Input: part model. Units: mm. Frame: model coordinates. Coordinates: 2 decimals unless noted, no trailing zeros. Order: outer loops, then holes, each group sorted by start corner. A loop starts at its lowest first (then second) coordinate and runs counter-clockwise, first axis right, second up. Notation, with made-up numbers: (-16, 7) -> (16, 7) arc R28 ccw to (16, 29) -> close; hole circle Ø1 at (83, 83). An arc over 180 degrees is marked (long way). One line per question, with ' | ' between items.
Autodesk Fusion 360 part; units mm, degrees
sketch "Sketch1" plane through (0, 0, 0) normal (0, 1, 0) x (1, 0, 0)
  circle A0 centre (0, 0) radius 1.55
  circle A1 centre (0, 0) radius 2.75
  line L0 (0, 2.75) -> (37, 2.75)
  line L1 (29.0028, 0) -> (29.0028, 0)
  line L2 (37, -2.75) -> (0, -2.75)
  arc A2 (39.75, 0) -> (37, 2.75) centre (37, 0) ccw
  arc A3 (37, -2.75) -> (39.75, 0) centre (37, 0) ccw
  dimension "d1" = 3.1
  dimension "d3" = 5.5
  dimension "d4" = 2.75
  dimension "d6" = 37
extrude "Extrude1" add sketch "Sketch1" along normal blind 2
equation "d6 = 40 mm - d4 - 0.25 mm"
1. Cut plane C-C, the plane z = 2. Return loops of the section in (x, y), and give its area (4 significant figures).
Recorded:
outline: (-1.89, 0) -> (38.89, 0) -> (38.89, 2) -> (-1.89, 2) -> close | area: 81.55 mm^2
2. Cut plane A-A, the plane z = 0. Return loops of the section in (x, y), and give its area (3 significant figures).
Recorded:
outline: (-2.75, 0) -> (-1.55, 0) -> (-1.55, 2) -> (-2.75, 2) -> close; (1.55, 0) -> (39.75, 0) -> (39.75, 2) -> (1.55, 2) -> close | area: 78.8 mm^2
3. Cut plane B-B, the plane y = 1.25. Return loops of the section in (x, z), and give its area (3 significant figures).
Recorded:
outline: (0, -2.75) -> (37, -2.75) arc R2.75 ccw to (37, 2.75) -> (0, 2.75) arc R2.75 ccw to start; hole circle Ø3.1 at (0, 0) | area: 220 mm^2
4. Ray query, line 1 (Z direction, x = 0, y = 0.6); line 2 (X direction, y = 0.6, z = 0); line 3 (X direction, y = 1.65, z = -0.55). Return the intervals inside material, ascending. Write a range as [from, to].
Recorded:
line 1: z = [-2.75, -1.55], [1.55, 2.75] | line 2: x = [-2.75, -1.55], [1.55, 39.75] | line 3: x = [-2.69, -1.45], [1.45, 39.69]
5. Mould query, pull axis Z, two halves, no side actions, for faces 1 (the face through (19, 1, 2.75)), 2 (the face through (-2.75, 0.99, 0.06)), 3 (the face through (18, 2, 0)), 4 (the face through (0.715, 0.986, -1.375)). Classes: released by +Z, released by -Z, zero draft, split by the parting line, or undercut.
Recorded:
face 1: released by +Z | face 2: split by the parting line | face 3: zero draft | face 4: undercut
